Here's the drawing with two shaded views (mm, measured from the low corner). I have some questions. A direction names the side the tool comes from. Give positions to 0.01 mm unless a question says otherwise; leave off trailing zeros. Write each loop counter-clockwise with the first axis right and the second up, starting at its lowest first coordinate (ties: lowest second). Pieces come first, ordered by that corner, then holes. Notation, with made-up numbers: (48.5, -13) -> (86.5, -13) arc R32 cw to (86.5, 26) -> close; hole circle Ø6 at (77, 73.5). An arc over 180 degrees is marked (long way). One line per question, with ' | ' between items.
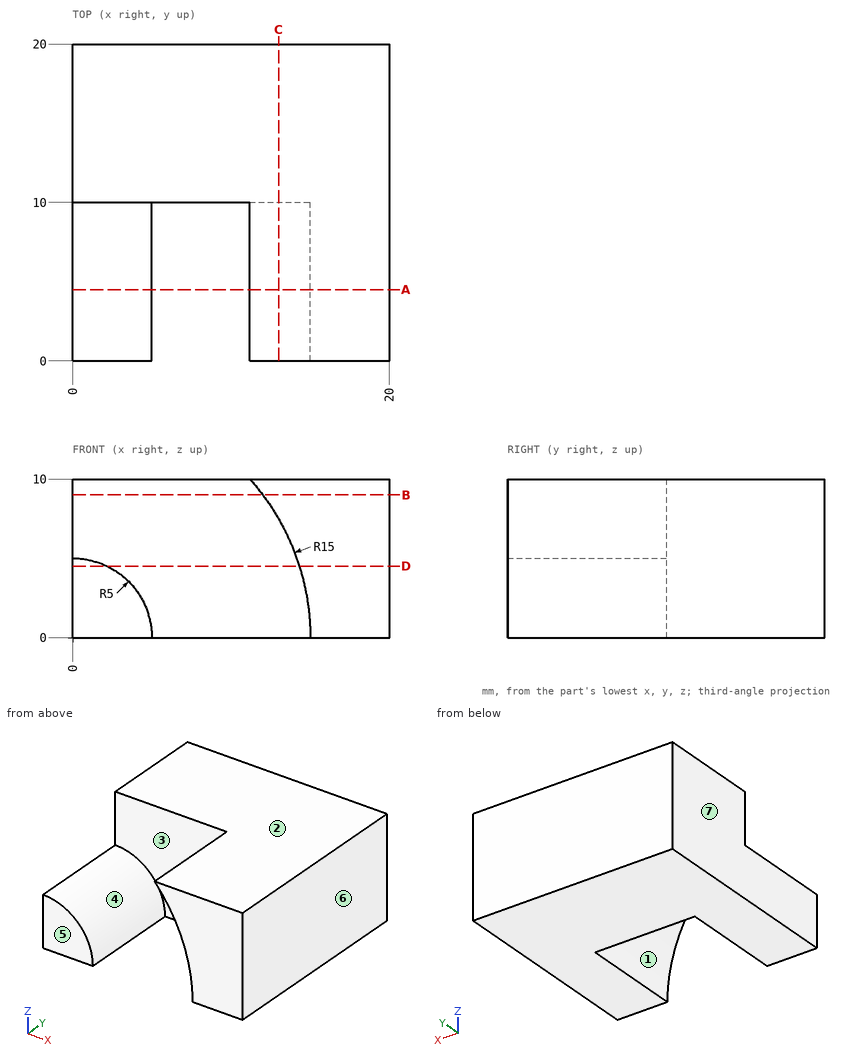
Q1. Will this pin go through, and if not, where does the flat tip stop? pin 1 (2 mm diameter, centred on x = 4, z = 6, fed in from -Y).
Answer below:
pin 1: stops at y = 10
Q2. Imagine slicing it at D-D on z = 4.5. Please give me the cut outline in (x, y).
Answer below:
outline: (0, 0) -> (2.18, 0) -> (2.18, 10) -> (14.31, 10) -> (14.31, 0) -> (20, 0) -> (20, 20) -> (0, 20) -> close
Q3. Imagine slicing it at B-B on z = 9. Please give me the cut outline in (x, y), and give its area (3 significant figures).
Answer below:
outline: (0, 10) -> (12, 10) -> (12, 0) -> (20, 0) -> (20, 20) -> (0, 20) -> close | area: 280 mm^2
Q4. Imagine slicing it at C-C on x = 13. Please give me the cut outline in (y, z).
Answer below:
outline: (0, 7.48) -> (10, 7.48) -> (10, 0) -> (20, 0) -> (20, 10) -> (0, 10) -> close
Q5. If I drill on line 1 along Y through (x, z) = (4.5, 5.75); line 2 along X through (y, z) = (3.25, 4); line 3 along X through (y, z) = (8.75, 1), over which ranges is the centre line in solid material (lowest first)?
Answer below:
line 1: y = 10 to 20 | line 2: x = 0 to 3, 14.46 to 20 | line 3: x = 0 to 4.9, 14.97 to 20
Q6. Imagine slicing it at A-A on y = 4.5. Please give me the cut outline in (x, z), and give its area (3 significant figures).
Answer below:
outline: (0, 0) -> (5, 0) arc R5 ccw to (0, 5) -> close; (11.18, 10) arc R15 cw to (15, 0) -> (20, 0) -> (20, 10) -> close | area: 81.6 mm^2
Q7. On a 3-axis mill with a long thin cutter (end or side, diameter ignored), from which of +Z, -Z, +X, -X, +Y, -Y can I reach the whole of each face in a straight line? I mean the marked faces 1, 2 and 3. Say none if no direction works.
Answer below:
face 1: -Z, -Y | face 2: +Z, +X, -X, +Y, -Y | face 3: -Y
Q8. If we mould it in two halves opening along X, with no side actions, what happens to the marked faces 4, 5, 6 and 7? For each: +X half, -X half, draft (parallel to the pull), parting line (faces both ways), or undercut.
Answer below:
face 4: undercut | face 5: draft | face 6: +X half | face 7: -X half
